Autodesk Inventor part; units mm, degrees
ref_plane "Work Plane1" through (39.9599, 0, 14.2875) normal (0, 0, 1) x (1, 0, 0)
ref_plane "YZ Plane" through (0, 0, 0) normal (1, 0, 0) x (0, 1, 0)
ref_plane "XZ Plane" through (0, 0, 0) normal (0, 1, 0) x (-1, 0, 0)
sketch "Sketch1" plane through (0, 0, 0) normal (0, 1, 0) x (-1, 0, 0)
  line L0 (38.1, 23.8125) -> (-38.1, 23.8125)
  line L1 (-38.1, 23.8125) -> (-38.1, -23.8125)
  line L2 (-38.1, -23.8125) -> (38.1, -23.8125)
  line L3 (38.1, -23.8125) -> (38.1, 23.8125)
  line L4 (38.1, 23.8125) -> (-38.1, -23.8125) construction
  line L5 (-38.1, 23.8125) -> (38.1, -23.8125) construction
  line L6 (0, 0) -> (-38.1, 0) construction
  line L7 (38.1, 30.1625) -> (-50.8, 30.1625)
  line L8 (-50.8, 30.1625) -> (-50.8, -30.1625)
  line L9 (-50.8, -30.1625) -> (38.1, -30.1625)
  line L10 (38.1, -30.1625) -> (38.1, 30.1625)
  line L11 (38.1, 30.1625) -> (-50.8, -30.1625) construction
  line L12 (-50.8, 30.1625) -> (38.1, -30.1625) construction
  point P0 (-6.35, 0)
  point P1 (38.1, 23.8125)
  dimension "d0" = 76.2
  dimension "d1" = 47.625
  dimension "d2" = 6.35
  dimension "d3" = 12.7
extrude "Extrusion1" add sketch "Sketch1" along normal blind 9.525 contours L0 L1 L2 L10 L9 L8 L7
chamfer "Chamfer1" distance 9.525 angle 45 2 edges at (50.8, 4.7625, 30.1625) (50.8, 4.7625, -30.1625)
fillet "Fillet1" radius 3.175 4 edges at (41.275, 4.7625, -30.1625) (50.8, 4.7625, -20.6375) (50.8, 4.7625, 20.6375) (41.275, 4.7625, 30.1625)
fillet "Fillet4" radius 3.175 2 edges at (38.1, 4.7625, -23.8125) (38.1, 4.7625, 23.8125)
sketch "Sketch2" plane through (50.8, 0, 19.3224) normal (1, 0, 0) x (0, 0, -1)
  line L0 (43.1349, 9.525) -> (-4.4901, 9.525)
  line L1 (43.1349, 0) -> (-4.4901, 0)
  circle A0 centre (19.3224, 4.7625) radius 3.175
  line L2 (0, 9.525) -> (38.6447, 9.525)
  line L3 (19.3224, 9.525) -> (19.3224, 0) construction
  line L4 (19.3224, 4.7625) -> (3.4474, 4.7625) construction
  circle A1 centre (3.4474, 4.7625) radius 1.7526
  circle A2 centre (35.1974, 4.7625) radius 1.7526
  point P0 (38.6447, 9.525)
  point P1 (6.35, 9.525)
  point P2 (38.6447, 0)
  point P3 (6.35, 0)
  dimension "d10" = 6.35
  dimension "d99" = 15.875
  dimension "d100" = 3.5052
  dimension "d103" = 360
extrude "Extrusion6" cut sketch "Sketch2" against normal through all
sketch "Sketch5" plane through (-38.1, 0, -30.1625) normal (0, 0, -1) x (-1, 0, 0)
  line L0 (0, 0) -> (0, 9.525)
  line L1 (0, 9.525) -> (-78.0599, 9.525)
  line L2 (-10.8754, 9.525) -> (-12.031, 6.35)
  line L3 (-12.031, 6.35) -> (-13.369, 6.35)
  line L4 (-13.369, 6.35) -> (-14.5246, 9.525)
  line L5 (-25.4, 9.525) -> (-25.4, 6.35) construction
  line L6 (0, 9.525) -> (0, 6.35) construction
  line L7 (-12.7, 9.525) -> (-12.7, 6.35) construction
  line L8 (-25.4, 7.9375) -> (0, 7.9375) construction
  line L9 (-15.8627, 9.525) -> (-17.0183, 6.35)
  line L10 (-17.0183, 6.35) -> (-18.3563, 6.35)
  line L11 (-18.3563, 6.35) -> (-19.5119, 9.525)
  line L12 (-17.6873, 9.525) -> (-17.6873, 6.35) construction
  line L13 (-20.8499, 9.525) -> (-22.0055, 6.35)
  line L14 (-22.0055, 6.35) -> (-23.3436, 6.35)
  line L15 (-23.3436, 6.35) -> (-24.4992, 9.525)
  line L16 (-22.6746, 9.525) -> (-22.6746, 6.35) construction
  line L17 (-25.8372, 9.525) -> (-26.9928, 6.35)
  line L18 (-26.9928, 6.35) -> (-28.3309, 6.35)
  line L19 (-28.3309, 6.35) -> (-29.4865, 9.525)
  line L20 (-27.6618, 9.525) -> (-27.6618, 6.35) construction
  line L21 (-30.8245, 9.525) -> (-31.9801, 6.35)
  line L22 (-31.9801, 6.35) -> (-33.3181, 6.35)
  line L23 (-33.3181, 6.35) -> (-34.4737, 9.525)
  line L24 (-32.6491, 9.525) -> (-32.6491, 6.35) construction
  line L25 (-35.8118, 9.525) -> (-36.9674, 6.35)
  line L26 (-36.9674, 6.35) -> (-38.3054, 6.35)
  line L27 (-38.3054, 6.35) -> (-39.461, 9.525)
  line L28 (-37.6364, 9.525) -> (-37.6364, 6.35) construction
  line L29 (-12.031, 6.35) -> (0, 6.35)
  line L30 (-5.8881, 9.525) -> (-7.0437, 6.35)
  line L31 (-8.3817, 6.35) -> (-9.5373, 9.525)
  line L32 (-8.9595, 7.9375) -> (0, 7.9375)
  point P0 (-38.1, 0)
  point P1 (-13.9468, 7.9375)
  point P2 (-11.4532, 7.9375)
  point P3 (-11.4532, 7.9375)
  point P4 (-16.4405, 7.9375)
  point P5 (-16.4405, 7.9375)
  point P6 (-4.9873, 6.35)
  point P7 (-30.3873, 6.35)
  point P8 (-18.9341, 7.9375)
  point P9 (-21.4277, 7.9375)
  point P10 (-21.4277, 7.9375)
  point P11 (-9.9746, 6.35)
  point P12 (-35.3746, 6.35)
  point P13 (-23.9214, 7.9375)
  point P14 (-26.415, 7.9375)
  point P15 (-26.415, 7.9375)
  point P16 (-14.9618, 6.35)
  point P17 (-40.3618, 6.35)
  point P18 (-28.9087, 7.9375)
  point P19 (-31.4023, 7.9375)
  point P20 (-31.4023, 7.9375)
  point P21 (-19.9491, 6.35)
  point P22 (-45.3491, 6.35)
  point P23 (-33.8959, 7.9375)
  point P24 (-36.3896, 7.9375)
  point P25 (-36.3896, 7.9375)
  point P26 (-24.9364, 6.35)
  point P27 (-50.3364, 6.35)
  point P28 (-38.8832, 7.9375)
  point P29 (-15.8627, 9.525)
  point P30 (-35.8118, 9.525)
  point P31 (-30.8245, 9.525)
  point P32 (-25.8372, 9.525)
  point P33 (-29.4865, 9.525)
  point P34 (-20.8499, 9.525)
  point P35 (-24.4992, 9.525)
  point P36 (-6.4659, 7.9375)
  point P37 (-6.4659, 7.9375)
  point P38 (0, 7.9375)
  point P39 (-9.5373, 9.525)
  dimension "d68" = 3.175
  dimension "d70" = 70
  dimension "d71" = 2.4936
  dimension "d74" = 4.9873
  dimension "d79" = 12.7
  dimension "d82" = 4.9873
extrude "Extrusion8" cut sketch "Sketch5" against normal through all contours L25 L26 L27 L1 | L21 L22 L23 L1 | L17 L18 L19 L1 | L13 L14 L15 L1 | L9 L10 L11 L1 | L32 L30 L1 L0 | L32 L31 L1 L30 | L3 L4 L1 L2
fillet "Fillet5" radius 1.5875 2 edges at (-29.1405, 7.9375, -26.9875) (-29.1405, 7.9375, 26.9875)
chamfer "Chamfer3" distance 1.5875 angle 45 2 edges at (-38.1, 7.9375, -26.9875) (-38.1, 7.9375, 26.9875)
chamfer "Chamfer4" distance 1.5875 angle 45 2 edges at (-38.1, 0, -26.9875) (-38.1, 0, 26.9875)
ref_plane "Work Plane1" through (39.9599, 0, 14.2875) normal (0, 0, 1) x (1, 0, 0)
sketch "Sketch7" plane through (39.9599, 0, 14.2875) normal (0, 0, 1) x (1, 0, 0)
  line L0 (0, 0) -> (-76.4724, 0)
  line L1 (-1.8599, 9.525) -> (-1.8599, 0)
  line L2 (-1.8599, 0) -> (4.4901, 0)
  line L3 (4.4901, 0) -> (4.4901, 2.3813) construction
  line L4 (4.4901, 2.3813) -> (-1.8599, 2.3812) construction
  line L5 (-1.8599, 2.3812) -> (-1.8599, 0)
  line L6 (-1.8599, 2.3812) -> (4.4901, 0)
  point P0 (-39.9599, 0)
  point P1 (-1.8599, 2.3812)
  dimension "d114" = 6.35
  dimension "d115" = 2.3813
extrude "Extrusion10" cut sketch "Sketch7" against normal blind 9.525
mirror "Mirror2" about plane through (0, 0, 0) normal (0, 0, 1) of "Extrusion10"
equation "\"d74\" = 1.5708 * d68"
equation "\"d82\" = d74"
equation "\"d69\" = 1.5708 * d68"
properties part number "Rack" material "Aluminum 6061"
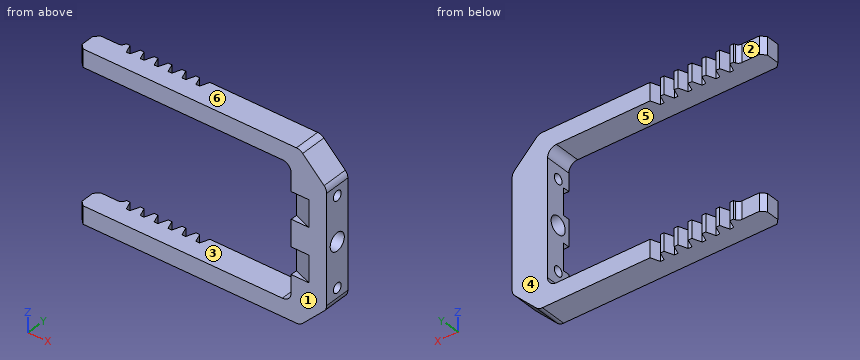
Input: part model. Units: mm. Frame: model coordinates. Face numbers are marked on the shaded views. A direction names the side the tool comes from. Round coordinates to 2 decimals unless told otherwise and drop trailing zeros. Write each loop counter-clockwise with the first axis right and the second up, starting at its lowest first coordinate (ties: lowest second). Pieces come first, ordered by that corner, then holes.
1) Cut plane A-A (z = 0). Return the cut outline in (x, y) (1 decimal).
2) Draft query along Z for the marked faces 4, 5 and 6. Return one class per face: pulls with the +Z half, pulls with the -Z half, needs draft (parallel to the pull), parting line crosses it, or undercut.
3) Cut plane C-C (z = -13). Return the cut outline in (x, y) (3 decimals), then the cut area to 3 significant figures.
4) Reachability of the marked faces 1, 2 and 3 from +Z, -Z, +X, -X, +Y, -Y: full face, straight path, thin tool, end or side. Return the list, or none.
5) Ray query, L1, parallel to Z at x = 35, y = 9; L2, parallel to X at y = 9.25, z = 7.5; L3, parallel to Y at x = -21, z = -27. Return the intervals inside material, ascending.
6) Contact query for flat-ended pins moving along their axis: P1, Ø1.2, axis at x = 42, y = 0.5, coming from the -Z side; P2, Ø0.7, axis at x = -0.5, z = 28.5, coming from the +Y side; P3, Ø5, axis at y = 3.5, z = 1, coming from the +X side; P4, Ø1.5, axis at y = 6.5, z = 1.5, coming from the +X side. Output: stop coordinate, or through.
7) Cut plane B-B (x = 33). Return the cut outline in (y, z) (1 decimal), then the cut area to 3 significant figures.
Geometry says:
1. outline: (38.1, 0) - (50.8, 0) - (50.8, 1.6) - (38.1, 1.6) - close; (38.1, 7.9) - (50.8, 7.9) - (50.8, 9.5) - (38.1, 9.5) - close
2. face 4: needs draft
2. face 5: undercut
2. face 6: pulls with the +Z half
3. outline: (38.1, 2.381) - (44.45, 0) - (50.8, 0) - (50.8, 9.525) - (38.1, 9.525) - close
3. area: 113 mm2
4. face 1: +Z, -Z, +X, -X, -Y
4. face 2: +Z, -Z, -X, +Y
4. face 3: -X, +Y, -Y
5. L1: z = -30.16 to -23.81, 23.81 to 30.16
5. L2: x = 38.1 to 50.8
5. L3: y = 0 to 6.35
6. P1: stops at z = -29.82
6. P2: stops at y = 6.35
6. P3: stops at x = 50.8
6. P4: passes through
7. outline: (0, -30.2) - (9.5, -30.2) - (9.5, -23.8) - (0, -23.8) - close; (0, 23.8) - (9.5, 23.8) - (9.5, 30.2) - (0, 30.2) - close
7. area: 121 mm2
